Model file for the job. Use its own axes, mm. Round coordinates to 2 decimals unless told otherwise and drop trailing zeros. Write each loop counter-clockwise with the first axis right and the second up, starting at its lowest first coordinate (ties: lowest second). Pieces come first, ordered by that corner, then holes.
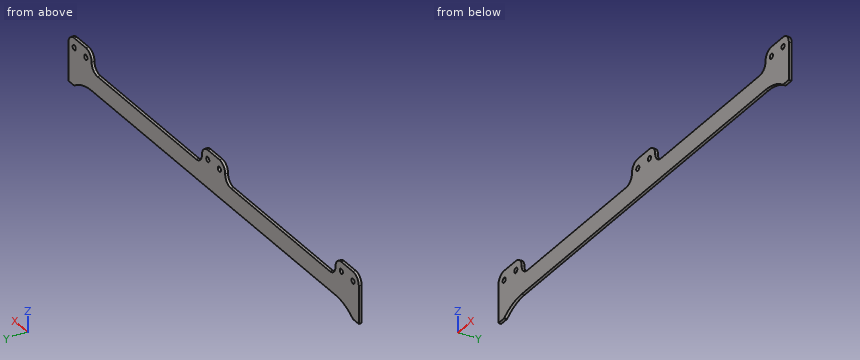
```python
from build123d import *

# Parameters (mm, degrees)
EXTRUDE_1_DEPTH        = 3
SKETCH_2_W             = 40
SKETCH_2_H             = 20
EXTRUDE_2_DEPTH        = 3
HOLE_WIZARD_M51_D      = 5.3
PATTERN_LINEAR_1_COUNT = 3
PATTERN_LINEAR_1_PITCH = 230
FILLET_1_R             = 10


with BuildPart() as part:
    # Эскиз1 → Бобышка-Вытянуть1 (new body)
    with BuildSketch(Plane(origin=(0, 0, 0), x_dir=(1, 0, 0), z_dir=(0, 1, 0))):
        with BuildLine():
            Line((210, 5), (-210, 5))
            ThreePointArc((-210, 5), (-225.811388301, 7.565835097), (-240, 15))
            Line((-240, 15), (-250, 15))
            Line((-250, 15), (-250, -15))
            Line((-250, -15), (250, -15))
            Line((250, -15), (250, 15))
            Line((250, 15), (240, 15))
            ThreePointArc((240, 15), (225.811388301, 7.565835097), (210, 5))
        make_face()
    extrude(amount=EXTRUDE_1_DEPTH)

    # Эскиз2 → Бобышка-Вытянуть2 (add)
    with BuildSketch(Plane(origin=(0, 3, 0), x_dir=(1, 0, 0), z_dir=(0, 1, 0))):
        with Locations((230, -25)):
            Rectangle(SKETCH_2_W, SKETCH_2_H)
    extrude_2 = extrude(amount=-EXTRUDE_2_DEPTH)

    # Отверстие с зазором M51 (through all)
    with Locations(Plane(origin=(0, 3, 0), x_dir=(1, 0, 0), z_dir=(0, 1, 0))):
        with Locations((220, -25), (240, -25)):
            hole_wizard_m51 = Hole(HOLE_WIZARD_M51_D / 2)

    # Линейный массив1: Бобышка-Вытянуть2, Отверстие с зазором M51 ×3
    with Locations(*[(-i * PATTERN_LINEAR_1_PITCH, 0, 0) for i in range(1, PATTERN_LINEAR_1_COUNT)]):
        add(extrude_2)
        add(hole_wizard_m51, mode=Mode.SUBTRACT)

    # Скругление1
    fillet_1_edges = [part.edges().sort_by_distance(p)[0] for p in [
        (-250, 1.5, 35),
        (-210, 1.5, 35),
        (-210, 1.5, 15),
        (-20, 1.5, 15),
        (-20, 1.5, 35),
        (20, 1.5, 35),
        (20, 1.5, 15),
        (210, 1.5, 15),
        (250, 1.5, 35),
        (210, 1.5, 35),
    ]]
    fillet(fillet_1_edges, radius=FILLET_1_R - 0.0001)  # a hair under: the kernel refuses the full size


solid = part.part
```
1) Cut at B-B on x = 59.5. List the corners of the cut face in (y, z), and give its area (3 significant figures).
2) Flat gauge pins, fed straight in: pin 1 Ø1.5 at (x, y) = (-144, 1) entering from +Z; pin 2 Ø3 at (x, z) = (10, 25) entering from -Y. Where does each tip first touch, or does it go through?
3) Wall check: probe 1 along X at (y, z) = (2.2, 31); probe 2 along X at (y, z) = (1.95, 28.5); probe 3 along Z at (x, y) = (172.5, 0.35). Give the ranges that are in metal, low to high.
4) Cut at A-A on y = 1.5. Give the number of separate pieces and of enclosed holes in the cut face, and give its area (3 significant figures).
Result sheet:
1. outline: (0, -5) - (3, -5) - (3, 15) - (0, 15) - close
1. area: 60.0 mm2
2. pin 1: stops at z = 15
2. pin 2: passes through
3. probe 1: x = -248 to -212, -18 to 18, 212 to 248
3. probe 2: x = -249.37 to -210.63, -19.37 to 19.37, 210.63 to 249.37
3. probe 3: z = -5 to 15
4. separate pieces: 1
4. enclosed holes: 6
4. area: 12,600 mm2
